Work out the finished part from the listing and answer in its coordinate system (mm). Round coordinates to 2 decimals unless told otherwise and drop trailing zeros. Order: outer loops, then holes, each group sorted by start corner. A loop starts at its lowest first (then second) coordinate and runs counter-clockwise, first axis right, second up. Notation, with made-up numbers: (30, 70.5) -> (63, 70.5) arc R7 ccw to (63, 82.5) -> close; hole circle Ø6 at (34.25, 66). An arc over 180 degrees is marked (long way). Use a Markdown table: item, result. Add a question column.
Item 1: A cutting plane is placed at B-B, the plane y = -167. Determine the outline of the cut face in (x, z).
Item 2: A cutting plane is placed at A-A, the plane x = -128. Determine the outline of the cut face in (y, z).
Item 3: Find the intervals of material crossed by L1, parallel to Z at x = 361.5, y = -753.5, in increasing order. Write a range as [from, to].
Item 4: Flat-ended cylindrical pins translate along their axes: P1, Ø12, axis at x = 47, y = -357.5, coming from the +Z side; P2, Ø3, axis at x = 35, y = -946.5, coming from the -Z side. Find the tip coordinate at first contact, or state that the pin passes through.
from build123d import *

# Parameters (mm, degrees)
CROQUIS1_W              = 850
CROQUIS1_H              = 1250
SALIENTE_EXTRUIR1_DEPTH = 300
CROQUIS3_R              = 2.5


with BuildPart() as part:
    # Croquis1 → Saliente-Extruir1 (new body)
    with BuildSketch(Plane.XY):
        with Locations((0, -555)):
            Rectangle(CROQUIS1_W, CROQUIS1_H)
    extrude(amount=SALIENTE_EXTRUIR1_DEPTH)

    # Barrer1: sweep along a path in Croquis2
    with BuildLine(Plane(origin=(0, 0, 0), x_dir=(1, 0, 0), z_dir=(0, 1, 0))) as barrer1_path:
        Line((-50, -300), (-50, -330))
        ThreePointArc((-50, -330), (-45.606601718, -340.606601718), (-35, -345))
        Line((-35, -345), (35, -345))
        ThreePointArc((35, -345), (45.606601718, -340.606601718), (50, -330))
        Line((50, -330), (50, -300))
    # Croquis3 → Barrer1 (sweep)
    with BuildSketch(Plane.XY.offset(300)):
        with Locations((-50, 0)):
            Circle(CROQUIS3_R)
    sweep(path=barrer1_path.line)


solid = part.part
Reported:
| question | item | result |
|---|---|---|
| 1 | outline | (-425, 0) -> (425, 0) -> (425, 300) -> (-425, 300) -> close |
| 2 | outline | (-1180, 0) -> (70, 0) -> (70, 300) -> (-1180, 300) -> close |
| 3 | L1 | [0, 300] |
| 4 | P1 | z = 300 |
| 4 | P2 | z = 0 |
